Design review of the part built by this model. Coordinates are the model's own, in mm. Coordinates: 2 decimals unless noted, no trailing zeros. Write each loop counter-clockwise with the first axis right and the second up, starting at its lowest first coordinate (ties: lowest second). Pieces come first, ordered by that corner, then holes. Notation, with made-up numbers: (11.25, 30) - (45.25, 30) arc R17 cw to (45.25, 40) - close; hole circle Ø1 at (14, 74.5). An arc over 180 degrees is marked (long way). Answer as CSV lines item,"result". Start each with the question number.
Q1. We need section C-C (x = 3). Write out the cut boundary in (y, z), plus the area to 3 significant figures.
Q2. We need section D-D (y = 0). Write out the cut boundary in (x, z), plus the area to 4 significant figures.
Q3. For line 1 along X through (y, z) = (283, 31); line 2 along Z through (x, y) = (31.5, 336.5); line 3 along Y through (x, z) = (-34.5, 0), list the stretches that pass through material, from the lowest coordinate up. Write a range as [from, to].
Q4. Clearance check with flat-ended pins moving along their axes: pin 1 (3 mm diameter, centred on x = -1, z = -44, fed in from +Y); pin 2 (22.5 mm diameter, centred on y = 2, z = 8, fed in from -X). State where each tip first meets the part, or that it passes through.
Q5. We need section A-A (y = 299.5). Write out the cut boundary in (x, z).
Q6. We need section B-B (z = 0). Write out the cut boundary in (x, y), plus the area to 4 significant figures.
from build123d import *

# Parameters (mm, degrees)
SKETCH1_W           = 100
SKETCH1_H           = 125
BOSS_EXTRUDE1_DEPTH = 500
SKETCH2_R           = 22.5
CUT_EXTRUDE1_DEPTH  = 25
CUT_EXTRUDE2_START  = -25
SKETCH3_R           = 22.5
CUT_EXTRUDE2_DEPTH  = 25
SKETCH4_W           = 65
SKETCH4_H           = 100
CUT_EXTRUDE3_DEPTH  = 400


with BuildPart() as part:
    # Sketch1 → Boss-Extrude1 (new, symmetric)
    with BuildSketch(Plane(origin=(0, 0, 0), x_dir=(1, 0, 0), z_dir=(0, 1, 0))):
        Rectangle(SKETCH1_W, SKETCH1_H)
    extrude(amount=BOSS_EXTRUDE1_DEPTH, both=True)

    # Sketch2 → Cut-Extrude1 (cut)
    with BuildSketch(Plane(origin=(50, 0, 0), x_dir=(0, 0, -1), z_dir=(1, 0, 0))):
        Circle(SKETCH2_R)
    extrude(amount=-CUT_EXTRUDE1_DEPTH, mode=Mode.SUBTRACT)

    # Sketch3 → Cut-Extrude2 (cut)
    with BuildSketch(Plane.ZY.offset(50).offset(CUT_EXTRUDE2_START)):
        with Locations(Location((0, 0, 0), (0, 0, 180))):
            Circle(SKETCH3_R)
    extrude(amount=CUT_EXTRUDE2_DEPTH, mode=Mode.SUBTRACT)

    # Sketch4 → Cut-Extrude3 (cut)
    with BuildSketch(Plane(origin=(0, 500, 0), x_dir=(1, 0, 0), z_dir=(0, 1, 0))):
        Rectangle(SKETCH4_W, SKETCH4_H)
    extrude(amount=-CUT_EXTRUDE3_DEPTH, mode=Mode.SUBTRACT)


solid = part.part
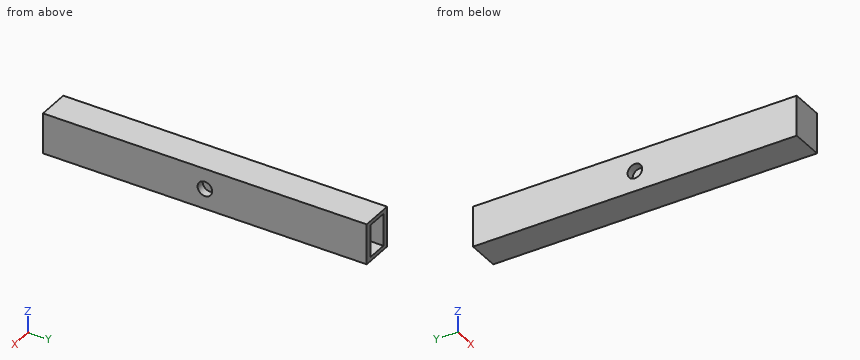
Results list:
1,outline,"(-500, -62.5) - (500, -62.5) - (500, -50) - (100, -50) - (100, 50) - (500, 50) - (500, 62.5) - (-500, 62.5) - close"
1,area,"85,000 mm2"
2,outline,"(-50, -62.5) - (50, -62.5) - (50, -22.5) - (25, -22.5) - (25, 22.5) - (50, 22.5) - (50, 62.5) - (-50, 62.5) - (-50, 22.5) - (-25, 22.5) - (-25, -22.5) - (-50, -22.5) - close"
2,area,"10,250 mm2"
3,line 1,"x = [-50, -32.5], [32.5, 50]"
3,line 2,"z = [-62.5, -50], [50, 62.5]"
3,line 3,"y = [-500, -22.5], [22.5, 500]"
4,pin 1,"stops at y = 100"
4,pin 2,"stops at x = -25"
5,outline,"(-50, -62.5) - (50, -62.5) - (50, 62.5) - (-50, 62.5) - close; hole (-32.5, -50) - (32.5, -50) - (32.5, 50) - (-32.5, 50) - close"
6,outline,"(-50, -500) - (50, -500) - (50, -22.5) - (25, -22.5) - (25, 22.5) - (50, 22.5) - (50, 500) - (32.5, 500) - (32.5, 100) - (-32.5, 100) - (-32.5, 500) - (-50, 500) - (-50, 22.5) - (-25, 22.5) - (-25, -22.5) - (-50, -22.5) - close"
6,area,"71,750 mm2"
